The model under review builds one solid part; all positions refer to its coordinate system, in mm. A direction names the side the tool comes from. Round coordinates to 2 decimals unless told otherwise and drop trailing zeros. Loops run counter-clockwise (first coordinate to the right, second up) from the corner with the lowest first, then second, coordinate; pieces in that order, holes last. Notation, with made-up numbers: M 84,84.25 L 124,84.25 A28 ccw 124,109.25 Z; hole C 20.5,59.5 d8. An arc over 180 degrees is marked long. Return JSON: item names as keys, results as strings. Group by question number.
Q1. To check wall thickness, follow line 1 along X through (y, z) = (0.05, 3.75); line 2 along X through (y, z) = (0, -3); line 3 along Z through (x, y) = (-8, 0.3). State the ranges of each line that lie inside material, in increasing order.
Q2. Consider section B-B (x = -9.5). State the section outline as (y, z) points.
Q3. Consider section C-C (z = -4.75). State the section outline as (x, y) points, and give its area (3 significant figures).
Q4. Consider section A-A (y = 0). State the section outline as (x, z) points.
Q5. For faces 1 (the face through (13.5, 0, -6)), 2 (the face through (0.175, 0.488, -0.108)), 3 (the face through (13, 0, -4)), 4 (the face through (-14, 0, 2)), list the 3-axis set-ups (+Z, -Z, +X, -X, +Y, -Y) from which the entire face can be reached by the end or side of a thin tool; tool diameter is ignored.
from build123d import *

# Parameters (mm, degrees)
F0_W      = 0.5
F0_H      = 1
F1_FACE_R = 0.5


with BuildPart() as f1:
    # F0 (on Front) → F1 (revolve)
    with BuildSketch(Plane.XZ):
        with Locations((-13.25, 3.5)):
            Rectangle(F0_W, F0_H)
    revolve(axis=Axis((-13.5, 0, 3.5), (0, 0, 1)))

    # F2: sweep along a path in F0
    with BuildLine(Plane.XZ) as f2_path:
        Line((-13.5, 3), (-13.5, 1))
        ThreePointArc((-13.5, 1), (-13.2071067812, 0.2928932188), (-12.5, 0))
        Line((-12.5, 0), (12.5, 0))
        ThreePointArc((12.5, 0), (13.2071067812, -0.2928932188), (13.5, -1))
        Line((13.5, -1), (13.5, -6))
    # F1_face (on face) → F2 (sweep)
    with BuildSketch(Plane(origin=(-13.5, 0, 3), x_dir=(1, 0, 0), z_dir=(0, 0, -1))):
        Circle(F1_FACE_R)
    sweep(path=f2_path.line)


solid = f1.part
Values:
{
 "1": {"line 1": "x = -14 to -13", "line 2": "x = 13 to 14", "line 3": "z = -0.4 to 0.4"},
 "2": {"outline": "C 0,0 d1"},
 "3": {"outline": "C 13.5,0 d1", "area": "0.785 mm2"},
 "4": {"outline": "M -14,1 A1.5 ccw -12.5,-0.5 L 12.5,-0.5 A0.5 cw 13,-1 L 13,-6 L 14,-6 L 14,-1 A1.5 ccw 12.5,0.5 L -12.5,0.5 A0.5 cw -13,1 L -13,4 L -14,4 Z"},
 "5": {"face 1": "-Z, +X, -X, +Y, -Y", "face 2": "none", "face 3": "-Z", "face 4": "+Z"}
}
